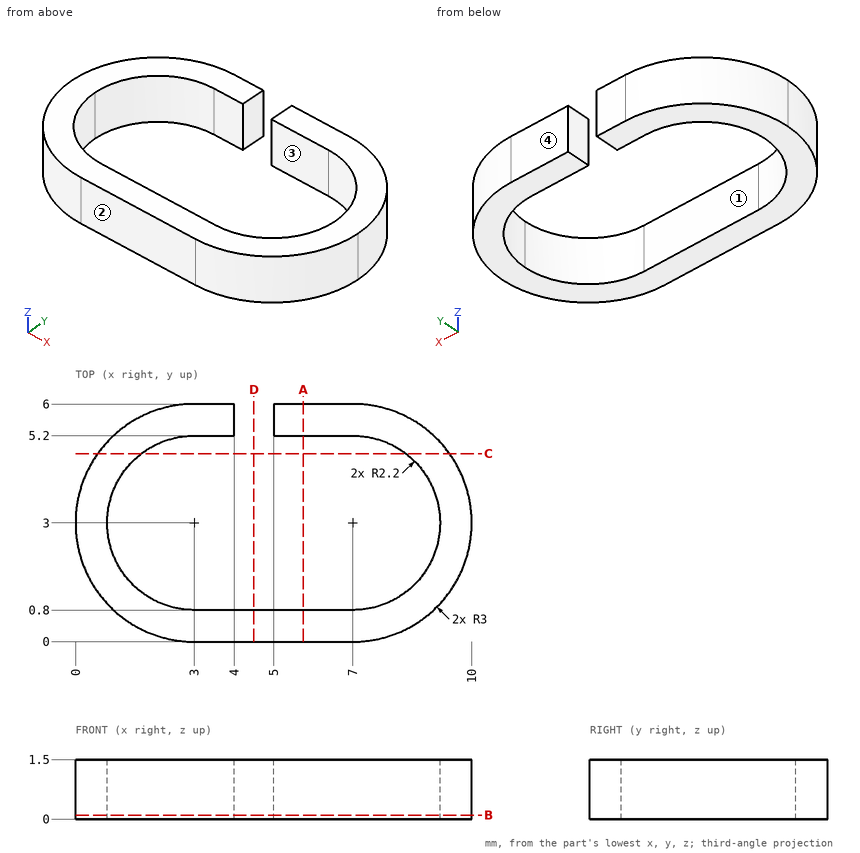
For this review, use the dimensioned drawing (mm, ordinates from the lowest corner) and the shaded views. A direction names the side the tool comes from. Coordinates: 2 decimals unless noted, no trailing zeros. Loops run counter-clockwise (first coordinate to the right, second up) from the corner with the lowest first, then second, coordinate; pieces in that order, holes last.
1. For the marked faces 1 and 2, list the 3-axis set-ups (+Z, -Z, +X, -X, +Y, -Y) from which the entire face can be reached by the end or side of a thin tool; tool diameter is ignored.
2. Mouldability with a two-part tool opening along X and no side actions: class the marked faces 3 and 4 as +X half, -X half, draft (parallel to the pull), parting line (faces both ways), or undercut.
3. Add section A-A, the plane x = 5.75. Give the boundary of the cut face in (y, z), then the cut area to 3 significant figures.
4. Add section D-D, the plane x = 4.5. Give the boundary of the cut face in (y, z).
5. For line 1 (Y direction, x = 5.25, z = 0.2); line 2 (X direction, y = 3, z = 0.85); line 3 (X direction, y = 5.5, z = 1), list the stretches that pass through material, from the lowest coordinate up.
6. Add section B-B, the plane z = 0.1. Give the boundary of the cut face in (x, y), then the cut area to 3 significant figures.
7. Add section C-C, the plane y = 4.75. Give the boundary of the cut face in (x, z).
8. Insertion check: P1, Ø0.6, axis at y = 5.5, z = 1, coming from the +X side. The pin has a flat end and moves straight along its axis. Give the tip position at first contact, or say it passes through.
Result:
1. face 1: +Z, -Z
1. face 2: +Z, -Z, +X, -X, -Y
2. face 3: undercut
2. face 4: draft
3. outline: (0, 0) - (0.8, 0) - (0.8, 1.5) - (0, 1.5) - close; (5.2, 0) - (6, 0) - (6, 1.5) - (5.2, 1.5) - close
3. area: 2.40 mm2
4. outline: (0, 0) - (0.8, 0) - (0.8, 1.5) - (0, 1.5) - close
5. line 1: y = 0 to 0.8, 5.2 to 6
5. line 2: x = 0 to 0.8, 9.2 to 10
5. line 3: x = 1.34 to 4, 5 to 8.66
6. outline: (0, 3) arc R3 ccw to (3, 0) - (7, 0) arc R3 ccw to (10, 3) arc R3 ccw to (7, 6) - (5, 6) - (5, 5.2) - (7, 5.2) arc R2.2 cw to (7, 0.8) - (3, 0.8) arc R2.2 cw to (3, 5.2) - (4, 5.2) - (4, 6) - (3, 6) arc R3 ccw to start
6. area: 18.7 mm2
7. outline: (0.56, 0) - (1.67, 0) - (1.67, 1.5) - (0.56, 1.5) - close; (8.33, 0) - (9.44, 0) - (9.44, 1.5) - (8.33, 1.5) - close
8. P1: stops at x = 9.04
